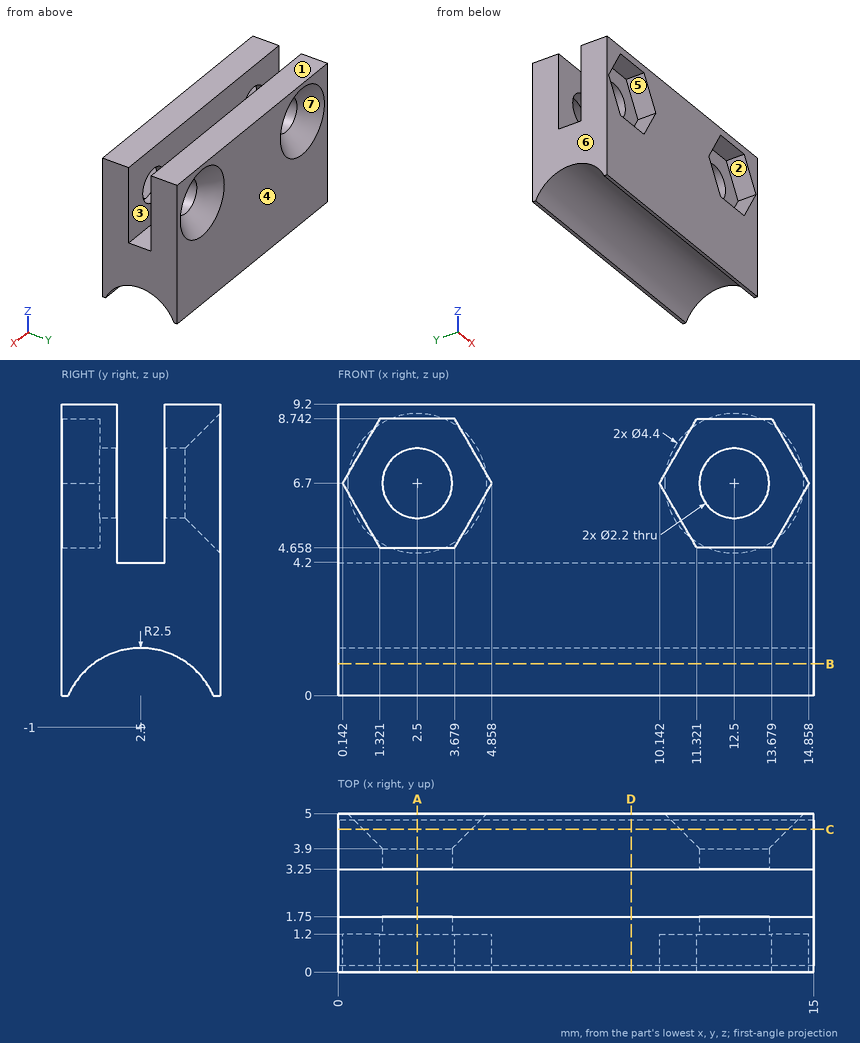
Can you work these out from the drawing? Everything is in mm from the part's minimum corner. A direction names the side the tool comes from. Coordinates: 2 decimals unless noted, no trailing zeros. Write each loop counter-clockwise with the first axis right and the second up, starting at its lowest first coordinate (ties: lowest second). Pieces come first, ordered by that corner, then holes. Notation, with made-up numbers: (76.5, 20.5) - (133.5, 20.5) arc R32 ccw to (133.5, 54.5) - close; hole circle Ø3 at (53, 32.25). An arc over 180 degrees is marked (long way). One line per item, written item: value.
1) On a 3-axis mill with a long thin cutter (end or side, diameter ignored), from which of +Z, -Z, +X, -X, +Y, -Y can I reach the whole of each face in a straight line? I mean the marked faces 1, 2 and 3. Say none if no direction works.
Model answer:
face 1: +Z, +X, -X, +Y, -Y
face 2: -Y
face 3: +Z, +X, -X
2) I need wall thicknesses on line 1 along X through (y, z) = (3.65, 6.7); line 2 along Y through (x, z) = (7, 5); line 3 along X through (y, z) = (4.1, 5.75). Which ranges of each line are inside material? Lowest first, please.
Model answer:
line 1: x = 0 to 1.4, 3.6 to 11.4, 13.6 to 15
line 2: y = 0 to 1.75, 3.25 to 5
line 3: x = 0 to 1.61, 3.39 to 11.61, 13.39 to 15
3) I'm going to push flat-ended pins straight in: P1, Ø4, axis at x = 10.5, z = 7.5, coming from the -Y side; P2, Ø3.5, axis at x = 12.5, z = 6.7, coming from the +Y side; P3, Ø2, axis at x = 11.5, z = 6.5, coming from the -Y side; P4, Ø3, axis at x = 12.5, z = 6.7, coming from the +Y side. Where does each tip first touch, or does it pass through?
Model answer:
P1: stops at y = 0
P2: stops at y = 4.55
P3: stops at y = 1.2
P4: stops at y = 4.3
4) Suppose I cut it at C-C on y = 4.5. Write out the boundary of the cut face in (x, z).
Model answer:
outline: (0, 0.5) - (15, 0.5) - (15, 9.2) - (0, 9.2) - close; hole circle Ø3.4 at (2.5, 6.7); hole circle Ø3.4 at (12.5, 6.7)
5) Suppose I cut it at D-D on x = 9.25. Write out the boundary of the cut face in (y, z).
Model answer:
outline: (0, 0) - (0.21, 0) arc R2.5 cw to (4.79, 0) - (5, 0) - (5, 9.2) - (3.25, 9.2) - (3.25, 4.2) - (1.75, 4.2) - (1.75, 9.2) - (0, 9.2) - close
6) Suppose I cut it at A-A on x = 2.5. Write out the boundary of the cut face in (y, z).
Model answer:
outline: (0, 0) - (0.21, 0) arc R2.5 cw to (4.79, 0) - (5, 0) - (5, 4.5) - (3.9, 5.6) - (3.25, 5.6) - (3.25, 4.2) - (1.75, 4.2) - (1.75, 5.6) - (1.2, 5.6) - (1.2, 4.66) - (0, 4.66) - close; (0, 8.74) - (1.2, 8.74) - (1.2, 7.8) - (1.75, 7.8) - (1.75, 9.2) - (0, 9.2) - close; (3.25, 7.8) - (3.9, 7.8) - (5, 8.9) - (5, 9.2) - (3.25, 9.2) - close
7) We'd pull the mould along X, two halves only. Please class the marked faces 4, 5, 6 and 7: pulls with the +X half, pulls with the -X half, needs draft (parallel to the pull), parting line crosses it, or undercut.
Model answer:
face 4: needs draft
face 5: undercut
face 6: pulls with the -X half
face 7: undercut
8) Suppose I cut it at B-B on z = 1. Write out the boundary of the cut face in (x, y).
Model answer:
outline: (0, 0) - (15, 0) - (15, 1) - (0, 1) - close; (0, 4) - (15, 4) - (15, 5) - (0, 5) - close
